Here's how the part is built. I have some questions about the finished solid (model axes, mm). Coordinates: 2 decimals unless noted, no trailing zeros. Loops run counter-clockwise (first coordinate to the right, second up) from the corner with the lowest first, then second, coordinate; pieces in that order, holes last.
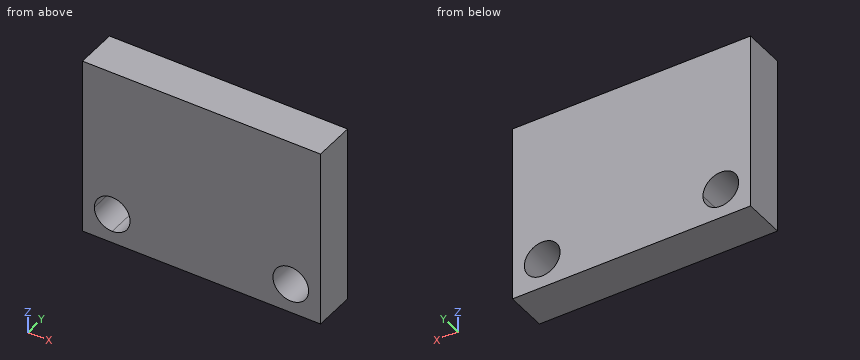
```python
from build123d import *

# Parameters (mm, degrees)
SKETCH1_W           = 10
SKETCH1_H           = 15
SKETCH1_R           = 1.5
BOSS_EXTRUDE1_DEPTH = 3.5


with BuildPart() as part:
    # Sketch1 → Boss-Extrude1 (new body)
    # profile 1 of 2: a face of its own
    with BuildSketch(Plane(origin=(0, 0, 0), x_dir=(1, 0, 0), z_dir=(0, 1, 0))):
        with Locations((15, 7.5)):
            Rectangle(SKETCH1_W, SKETCH1_H)
        with Locations(Location((17.5, 12.5, 0), (0, 0, 270))):
            Circle(SKETCH1_R, mode=Mode.SUBTRACT)
    # profile 2 of 2: a face of its own
    with BuildSketch(Plane(origin=(0, 0, 0), x_dir=(1, 0, 0), z_dir=(0, 1, 0))):
        with Locations((5, 7.5)):
            Rectangle(SKETCH1_W, SKETCH1_H)
        with BuildLine():
            ThreePointArc((1, 12.5), (1.439339828, 13.560660172), (2.5, 14))
            ThreePointArc((2.5, 14), (3.560660172, 13.560660172), (4, 12.5))
            ThreePointArc((4, 12.5), (2.5, 11), (1, 12.5))
        make_face(mode=Mode.SUBTRACT)
    extrude(amount=BOSS_EXTRUDE1_DEPTH)


solid = part.part
```
1. I want a section at D-D (x = 1.5). Please give me the cut outline in (y, z), then the cut area to 3 significant figures.
2. I want a section at B-B (x = 17.5). Please give me the cut outline in (y, z).
3. I want a section at A-A (y = 0.65). Please give me the cut outline in (x, z).
4. I want a section at C-C (z = -13.75). Please give me the cut outline in (x, y).
5. I need wall thicknesses on line 1 along X through (y, z) = (2.2, -12.5); line 2 along X through (y, z) = (1.05, -13). Which ranges of each line are inside material? Lowest first, please.
Response values:
1. outline: (0, -15) - (3.5, -15) - (3.5, -13.62) - (0, -13.62) - close; (0, -11.38) - (3.5, -11.38) - (3.5, 0) - (0, 0) - close
1. area: 44.7 mm2
2. outline: (0, -15) - (3.5, -15) - (3.5, -14) - (0, -14) - close; (0, -11) - (3.5, -11) - (3.5, 0) - (0, 0) - close
3. outline: (0, -15) - (20, -15) - (20, 0) - (0, 0) - close; hole circle Ø3 at (2.5, -12.5); hole circle Ø3 at (17.5, -12.5)
4. outline: (0, 0) - (1.67, 0) - (1.67, 3.5) - (0, 3.5) - close; (3.33, 0) - (16.67, 0) - (16.67, 3.5) - (3.33, 3.5) - close; (18.33, 0) - (20, 0) - (20, 3.5) - (18.33, 3.5) - close
5. line 1: x = 0 to 1, 4 to 16, 19 to 20
5. line 2: x = 0 to 1.09, 3.91 to 16.09, 18.91 to 20
